For this review, take the finished solid that the model builds, in its own axes (mm). Round coordinates to 2 decimals unless told otherwise and drop trailing zeros. Loops run counter-clockwise (first coordinate to the right, second up) from the corner with the lowest first, then second, coordinate; pieces in that order, holes last. Notation, with made-up numbers: M 32,-35.75 L 56,-35.75 A27 cw 56,-1.75 Z; hole C -24.5,41.5 d11. An arc over 180 degrees is marked long. One line per question, with ' | ' between items. Start each with the question number.
1) We need section C-C (y = -5). Give the boundary of the cut face in (x, z).
2) For probe 1 along Y at (x, z) = (13.5, -0.25); probe 2 along Y at (x, z) = (7.5, -0.85); probe 3 along Y at (x, z) = (6, -0.5), list the stretches that pass through material, from the lowest coordinate up. Write a range as from..to.
3) We need section D-D (z = -0.25). State how many separate pieces and enclosed holes the cut face has, and give its area (3 significant figures).
4) We need section B-B (x = 13.5). Give the boundary of the cut face in (y, z).
5) We need section A-A (y = -28.5). Give the boundary of the cut face in (x, z), and give its area (3 significant figures).
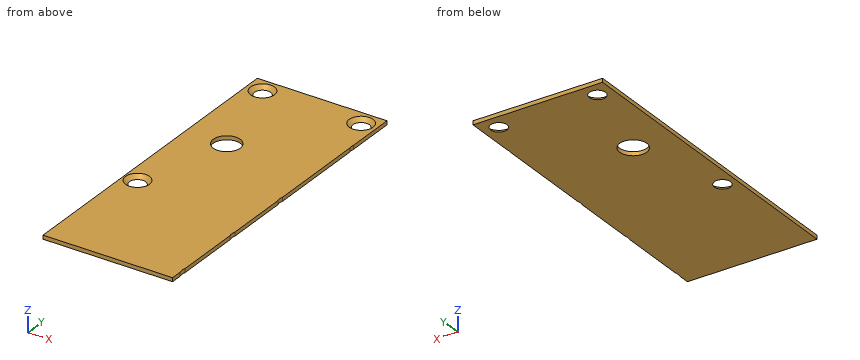
Autodesk Inventor part; units mm, degrees
ref_plane "YZ Plane" through (0, 0, 0) normal (1, 0, 0) x (0, 1, 0)
ref_plane "XZ Plane" through (0, 0, 0) normal (0, 1, 0) x (-1, 0, 0)
ref_plane "XY Plane" through (0, 0, 0) normal (0, 0, 1) x (1, 0, 0)
ref_plane "Work Plane1" through (3, 4, -1) normal (0, 0, 1) x (0, -1, 0)
sketch "Sketch1" plane through (3, 4, -1) normal (0, 0, 1) x (0, -1, 0)
  line L0 (87.75, 33.5) -> (84.9105, 33.5)
  line L1 (5, 0) -> (5, 33.5)
  line L2 (5, 0) -> (87.75, 0)
  line L3 (5, 0) -> (60, 0)
  line L4 (5, -3) -> (5, 0)
  line L5 (4, -3) -> (60, -3)
  line L6 (60, -3) -> (60, 0)
  line L7 (60, 0) -> (61.551, 0)
  circle A0 centre (74.375, 17.375) radius 6.75
  line L8 (60, 0) -> (60, 33.5)
  circle A1 centre (32.5, 10.5) radius 5.5
  circle A2 centre (9, 4) radius 2.1
  circle A3 centre (9, 29.5) radius 2.1
  circle A4 centre (56.5, 3.5) radius 2.1
  line L9 (82.9895, 33.5) -> (65.5855, 33.5)
  line L10 (63.6645, 33.5) -> (47.1605, 33.5)
  spline S0 degree 2 poles (47.1605, 33.5) (46.2, 33.2071) (45.2395, 33.5) knots 0 0 0 0.194422 0.194422 0.194422 weights 1 1.05 1
  line L11 (45.2395, 33.5) -> (19.3669, 33.5)
  spline S1 degree 2 poles (19.3669, 33.5) (18.6923, 33.3555) (18.0177, 33.5) knots 0 0 0 0.135703 0.135703 0.135703 weights 1 1.02375 1
  spline S2 degree 2 poles (84.9105, 33.5) (83.95, 33.2071) (82.9895, 33.5) knots 0 0 0 0.194422 0.194422 0.194422 weights 1 1.05 1
  spline S3 degree 2 poles (65.5855, 33.5) (64.625, 33.2071) (63.6645, 33.5) knots 0 0 0 0.194422 0.194422 0.194422 weights 1 1.05 1
  line L12 (87.75, 0) -> (87.75, 33.5)
  line L13 (18.0177, 33.5) -> (5, 33.5)
  arc A5 (60, 1.551) -> (61.551, 0) centre (62.75, 2.75) ccw
  line L14 (60, 1.551) -> (60, 0)
  point P0 (89.75, 33.5)
  point P1 (52, 0)
  point P2 (64.076, 0)
  point P3 (87.674, 0)
  point P4 (63.25, 3.25)
  point P5 (86.9105, 33.5)
  point P6 (84.9895, 33.5)
  point P7 (63.949, 0)
  point P8 (84.801, 0)
extrude "Extrusion1" add sketch "Sketch1" along normal blind 1 contours L12 L2 A5 L8 L10 S3 L9 S2 L0 | L2 L8 A5 | L2 L1 L13 S1 L11 S0 L10 L8 | A0 | A1 | A2 | A3 | A4
sketch "Sketch2" plane through (3, 4, 0) normal (0, 0, 1) x (1, 0, 0)
  line L0 (12.5287, -34.71) -> (8.4496, -34.6899)
  arc A0 (8.4713, -30.29) -> (8.4496, -34.6899) centre (10.5, -32.5) ccw
  line L1 (8.4713, -30.29) -> (12.5504, -30.3101)
  arc A1 (12.5287, -34.71) -> (12.5504, -30.3101) centre (10.5, -32.5) ccw
  circle A2 centre (10.5, -32.5) radius 3
  circle A3 centre (10.5, -32.5) radius 3.5
  point P0 (-3, -4)
  dimension "d5" = 0.5
extrude "Extrusion2" cut sketch "Sketch2" against normal up to next contours A2 L0 | L0 A0 L1 A1 | A2 L1 | A3
sketch "Sketch3" plane through (3, 4, 0) normal (0, 0, 1) x (1, 0, 0)
  circle A0 centre (10.5, -32.5) radius 3.5
  line L0 (0, -5) -> (0, -87.75)
  line L1 (33.5, -5) -> (0, -5)
  circle A1 centre (3.5, -56.5) radius 3.5
  circle A2 centre (4, -9) radius 4
  circle A3 centre (3.5, -56.5) radius 2.6
  circle A4 centre (4, -9) radius 2.6
  circle A5 centre (29.5, -9) radius 4
  circle A6 centre (29.5, -9) radius 2.6
  line L2 (33.5, -63.6645) -> (33.5, -47.1605)
  line L3 (33.5, -45.2395) -> (33.5, -19.3669)
  line L4 (33.5, -18.0177) -> (33.5, -5)
  line L5 (0, -87.75) -> (33.5, -87.75)
  line L6 (33.5, -87.75) -> (33.5, -84.9105)
  line L7 (33.5, -82.9895) -> (33.5, -65.5855)
  point P0 (-3, -4)
  dimension "d8" = 7
  dimension "d17" = 8
  dimension "d18" = 5.2
  dimension "d19" = 5.2
  dimension "d20" = 4
  dimension "d21" = 4
  dimension "d22" = 8
  dimension "d23" = 5.2
  dimension "d25" = 4
hole "Hole1" at (6.5, -52.5, 0) at (7, -5, 0) at (32.5, -5, 0) direction (0, 0, -1) diameter 3.6 end through all countersink diameter 6.2 countersink angle 90
properties part number "right_metal_gear_bracker"
Answers below:
1) outline: M 3,-1 L 4.9,-1 L 3.9,0 L 3,0 Z; M 9.1,-1 L 30.4,-1 L 29.4,0 L 10.1,0 Z; M 34.6,-1 L 36.5,-1 L 36.5,0 L 35.6,0 Z
2) probe 1: -83.75..-32, -25..-1 | probe 2: -83.75..-54.52, -50.48..-7.19, -2.81..-1 | probe 3: -83.75..-55.05, -49.95..-7.4, -2.6..-1
3) separate pieces: 1 | enclosed holes: 4 | area: 2,660 mm^2
4) outline: M -83.75,-1 L -32,-1 L -32,0 L -83.75,0 Z; M -25,-1 L -1,-1 L -1,0 L -25,0 Z
5) outline: M 3,-1 L 10,-1 L 10,0 L 3,0 Z; M 17,-1 L 36.5,-1 L 36.5,0 L 17,0 Z | area: 26.5 mm^2
